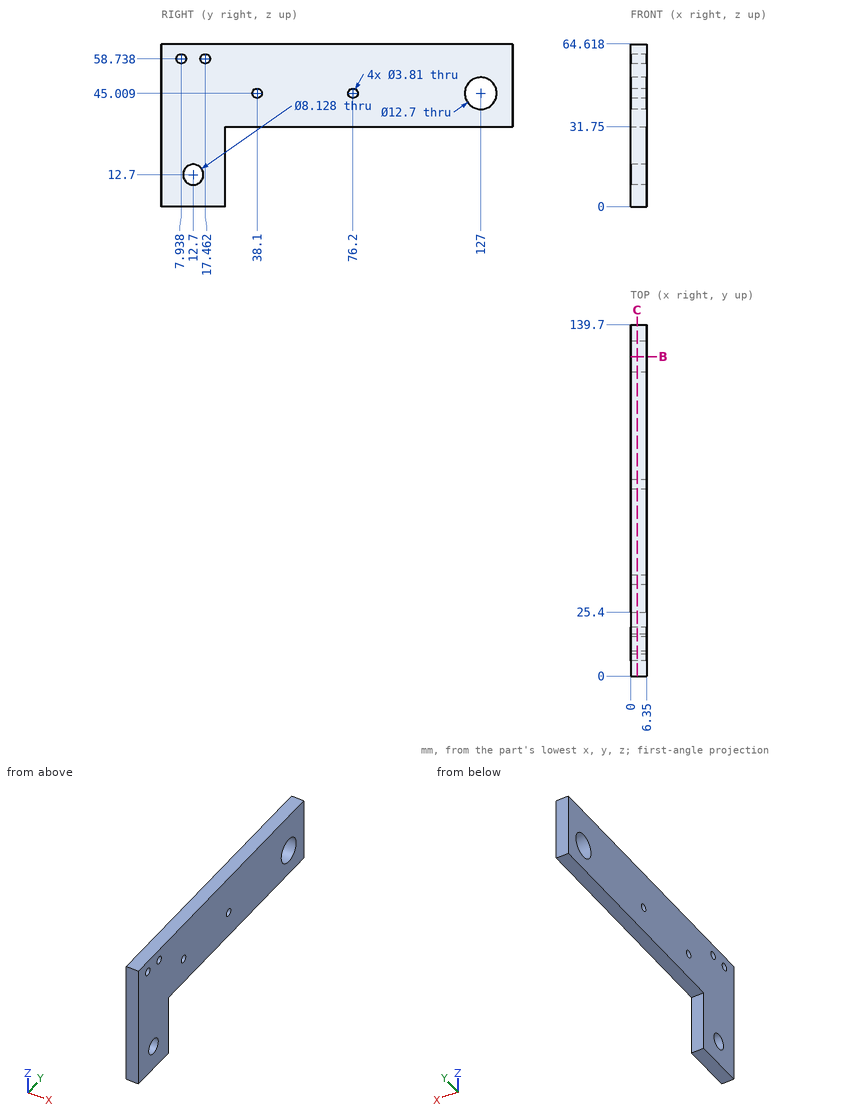
Here's the drawing with two shaded views (mm, measured from the low corner). I have some questions. Round coordinates to 2 decimals unless told otherwise and drop trailing zeros. Write each loop counter-clockwise with the first axis right and the second up, starting at its lowest first coordinate (ties: lowest second). Pieces come first, ordered by that corner, then holes. Notation, with made-up numbers: M 25,60 L 46,60 A20 ccw 46,84 Z; hole C -38.5,63 d2. An arc over 180 degrees is marked long. Answer in a Markdown table with one row per item. Add a question column.
Q1. Imagine slicing it at C-C (x = 2.5). Give the number of separate pieces and of enclosed holes in the cut face, then the cut area to 3 significant figures.
Q2. If I drill on line 1 (Z direction, x = 0.5, y = 46); line 2 (Y direction, x = 2.5, z = 26.5); line 3 (Z direction, x = 2.25, y = 13), over which ranges is the centre line in solid material (lowest first)? Write a range as from..to.
Q3. Imagine slicing it at B-B (y = 127). Please give me the cut outline in (x, z).
Q4. Will these pins go through, and if not, where does the flat tip stop? pin 1 Ø3.5 at (y, z) = (76.2, 45.01) entering from +X (1 decimal); pin 2 Ø3 at (x, z) = (3, 9) entering from +Y; pin 3 Ø1.5 at (x, y) = (4.5, 69) entering from -Z.
Values:
| question | item | result |
|---|---|---|
| 1 | separate pieces | 1 |
| 1 | enclosed holes | 6 |
| 1 | area | 5,170 mm^2 |
| 2 | line 1 | 31.75..64.62 |
| 2 | line 2 | 0..25.4 |
| 2 | line 3 | 0..8.65, 16.75..64.62 |
| 3 | outline | M 0,31.75 L 6.35,31.75 L 6.35,38.66 L 0,38.66 Z; M 0,51.36 L 6.35,51.36 L 6.35,64.62 L 0,64.62 Z |
| 4 | pin 1 | through |
| 4 | pin 2 | y = 25.4 |
| 4 | pin 3 | z = 31.75 |
